Design review of the part built by this model. Coordinates are the model's own, in mm. A direction names the side the tool comes from. Give positions to 0.01 mm unless a question says otherwise; leave off trailing zeros. Loops run counter-clockwise (first coordinate to the right, second up) from the corner with the lowest first, then second, coordinate; pieces in that order, holes last. Notation, with made-up numbers: (36, 59.25) - (71, 59.25) arc R6 ccw to (71, 66.25) - close; hole circle Ø6 at (84.25, 89.5). An arc over 180 degrees is marked (long way). Put each result on its own line as item: value. Start each with the question number.
```python
from build123d import *

# Parameters (mm, degrees)
EXTRUDE_1_DEPTH     = 80
CUT_EXTRUDE_1_DEPTH = 40
EXTRUDE_2_DEPTH     = 40
SKETCH_5_R          = 21.930814163
SKETCH_5_R_2        = 25.847454044
EXTRUDE_3_DEPTH     = 30
SKETCH_6_R          = 10
EXTRUDE_4_DEPTH     = 20


with BuildPart() as part:
    # 草图2 → 凸台-拉伸1 (new body)
    with BuildSketch(Plane(origin=(0, 0, 0), x_dir=(0, 0, -1), z_dir=(1, 0, 0))):
        with BuildLine():
            Line((158.264812498, -105.800263885), (278.081233304, -38.403527181))
            ThreePointArc((278.081233304, -38.403527181), (294.118007975, -22.634152676), (300, -0.925779085))
            Line((300, -0.925779085), (300, 0.925779085))
            ThreePointArc((300, 0.925779085), (287.405591591, 31.331370676), (257, 43.925779085))
            Line((257, 43.925779085), (-257, 43.925779085))
            ThreePointArc((-257, 43.925779085), (-287.405591591, 31.331370676), (-300, 0.925779085))
            Line((-300, 0.925779085), (-300, -0.925779085))
            ThreePointArc((-300, -0.925779085), (-294.118007975, -22.634152676), (-278.081233304, -38.403527181))
            Line((-278.081233304, -38.403527181), (-158.264812498, -105.800263885))
            ThreePointArc((-158.264812498, -105.800263885), (-139.316019316, -113.463120111), (-119.043913327, -116.074220915))
            Line((-119.043913327, -116.074220915), (119.043913327, -116.074220915))
            ThreePointArc((119.043913327, -116.074220915), (139.316019316, -113.463120111), (158.264812498, -105.800263885))
        make_face()
    extrude(amount=EXTRUDE_1_DEPTH)

    # 草图3 → 切除-拉伸1 (cut)
    with BuildSketch(Plane(origin=(80, 0, 0), x_dir=(0, 0, -1), z_dir=(1, 0, 0))):
        with BuildLine():
            Line((257, 33.925779085), (-257, 33.925779085))
            ThreePointArc((-257, 33.925779085), (-280.334523779, 24.260302864), (-290, 0.925779085))
            Line((-290, 0.925779085), (-290, -0.925779085))
            ThreePointArc((-290, -0.925779085), (-285.485913097, -17.585693701), (-273.178620908, -29.68777181))
            Line((-273.178620908, -29.68777181), (-153.362200102, -97.084508514))
            ThreePointArc((-153.362200102, -97.084508514), (-136.782006067, -103.789507712), (-119.043913327, -106.074220915))
            Line((-119.043913327, -106.074220915), (119.043913327, -106.074220915))
            ThreePointArc((119.043913327, -106.074220915), (136.782006067, -103.789507712), (153.362200102, -97.084508514))
            Line((153.362200102, -97.084508514), (273.178620908, -29.68777181))
            ThreePointArc((273.178620908, -29.68777181), (285.485913097, -17.585693701), (290, -0.925779085))
            Line((290, -0.925779085), (290, 0.925779085))
            ThreePointArc((290, 0.925779085), (280.334523779, 24.260302864), (257, 33.925779085))
        make_face()
    extrude(amount=-CUT_EXTRUDE_1_DEPTH, mode=Mode.SUBTRACT)

    # 草图4 → 凸台-拉伸2 (add)
    with BuildSketch(Plane(origin=(40, 0, 0), x_dir=(0, 0, -1), z_dir=(1, 0, 0))):
        with BuildLine():
            Line((-237.264786543, 20.974123526), (-239.546765639, 17.833248756))
            ThreePointArc((-239.546765639, 17.833248756), (-236.865961455, 14.739716181), (-234.683185749, 11.276748513))
            Line((-234.683185749, 11.276748513), (-230.908435146, 12.503239332))
            Line((-230.908435146, 12.503239332), (-228.206060722, 4.186186056))
            Line((-228.206060722, 4.186186056), (-231.89838046, 2.986478649))
            ThreePointArc((-231.89838046, 2.986478649), (-231.547897142, -1.09197894), (-231.817475826, -5.176582004))
            Line((-231.817475826, -5.176582004), (-228.042725222, -6.403072824))
            Line((-228.042725222, -6.403072824), (-230.745099646, -14.720126099))
            Line((-230.745099646, -14.720126099), (-234.437419384, -13.520418692))
            ThreePointArc((-234.437419384, -13.520418692), (-236.551129646, -17.025969117), (-239.170092825, -20.172028037))
            Line((-239.170092825, -20.172028037), (-236.837168653, -23.383022689))
            Line((-236.837168653, -23.383022689), (-243.912076745, -28.5232443))
            Line((-243.912076745, -28.5232443), (-246.194055841, -25.38236953))
            ThreePointArc((-246.194055841, -25.38236953), (-249.964594205, -26.976011679), (-253.932586961, -27.981838877))
            Line((-253.932586961, -27.981838877), (-253.932586961, -31.950846543))
            Line((-253.932586961, -31.950846543), (-262.677654297, -31.950846543))
            Line((-262.677654297, -31.950846543), (-262.677654297, -28.068511818))
            ThreePointArc((-262.677654297, -28.068511818), (-266.664803265, -27.141528556), (-270.466187231, -25.62293223))
            Line((-270.466187231, -25.62293223), (-272.799111403, -28.833926882))
            Line((-272.799111403, -28.833926882), (-279.874019495, -23.693705272))
            Line((-279.874019495, -23.693705272), (-277.592040399, -20.552830502))
            ThreePointArc((-277.592040399, -20.552830502), (-280.272844583, -17.459297927), (-282.455620289, -13.996330258))
            Line((-282.455620289, -13.996330258), (-286.230370892, -15.222821078))
            Line((-286.230370892, -15.222821078), (-288.932745316, -6.905767802))
            Line((-288.932745316, -6.905767802), (-285.240425578, -5.706060395))
            ThreePointArc((-285.240425578, -5.706060395), (-285.590908896, -1.627602806), (-285.321330213, 2.457000258))
            Line((-285.321330213, 2.457000258), (-289.096080816, 3.683491078))
            Line((-289.096080816, 3.683491078), (-286.393706392, 12.000544353))
            Line((-286.393706392, 12.000544353), (-282.701386654, 10.800836946))
            ThreePointArc((-282.701386654, 10.800836946), (-280.587676392, 14.306387371), (-277.968713213, 17.452446291))
            Line((-277.968713213, 17.452446291), (-280.301637385, 20.663440943))
            Line((-280.301637385, 20.663440943), (-273.226729293, 25.803662554))
            Line((-273.226729293, 25.803662554), (-270.944750197, 22.662787784))
            ThreePointArc((-270.944750197, 22.662787784), (-267.174211833, 24.256429933), (-263.206219077, 25.262257132))
            Line((-263.206219077, 25.262257132), (-263.206219077, 29.231264797))
            Line((-263.206219077, 29.231264797), (-254.461151741, 29.231264797))
            Line((-254.461151741, 29.231264797), (-254.461151741, 25.348930073))
            ThreePointArc((-254.461151741, 25.348930073), (-250.474002773, 24.42194681), (-246.672618807, 22.903350484))
            Line((-246.672618807, 22.903350484), (-244.339694635, 26.114345136))
            Line((-244.339694635, 26.114345136), (-237.264786543, 20.974123526))
        make_face()
    extrude(amount=EXTRUDE_2_DEPTH)

    # 草图5 → 凸台-拉伸3 (add)
    with BuildSketch(Plane(origin=(40, 0, 0), x_dir=(0, 0, -1), z_dir=(1, 0, 0))):
        with Locations((-129.354117612, -82.245801831)):
            Circle(SKETCH_5_R)
        with Locations((-44.354117612, -82.245801831)):
            Circle(SKETCH_5_R)
        with Locations((40.645882388, -82.245801831)):
            Circle(SKETCH_5_R)
        with Locations((125.645882388, -82.245801831)):
            Circle(SKETCH_5_R)
        with Locations((258.847706699, 0)):
            Circle(SKETCH_5_R_2)
    extrude(amount=EXTRUDE_3_DEPTH)

    # 草图6 → 凸台-拉伸4 (add)
    with BuildSketch(Plane.ZY):
        with Locations((-180, -16.074220915)):
            Circle(SKETCH_6_R)
        with Locations((180, -16.074220915)):
            Circle(SKETCH_6_R)
    extrude(amount=EXTRUDE_4_DEPTH)


solid = part.part
```
Item 1: Machinability: for faces 1 (the flat face through (39, -116.074, 2)), 2 (the cylindrical face through (-9.86, -19.9, 189.24)), 3 (the cylindrical face through (60.28, -103.853, -136.539)), which of the approach directions +Z, -Z, +X, -X, +Y, -Y give a long, thin tool a straight path to every point of the face, cutting with its end or side? Answer none if there is none.
Item 2: For L1, parallel to Y at x = 70, z = 102; L2, parallel to Y at x = 57.5, z = 259; L3, parallel to Z at x = -9.5, y = -17.5, list the stretches that pass through material, from the lowest coordinate up. Write a range as from..to.
Item 3: Consider section B-B (z = -246). State the section outline as (x, y) points.
Item 4: Consider section C-C (y = -76). State the section outline as (x, z) points.
Item 5: Consider section A-A (x = 34). State the section outline as (y, z) points, plus the area to 3 significant figures.
Item 6: For P1, Ø4.5, axis at x = 63, z = 256.5, coming from the -Y side; P2, Ø1.5, axis at y = -7, z = -44.5, coming from the -X side; P3, Ø4.5, axis at x = 51, z = 260, coming from the +Y side, all flat-tipped, find the tip position at first contact; note any pin that passes through.
Item 7: Mouldability with a two-part tool opening along Z and no side actions: class faces 4 (the flat face through (39.44, -71.63, 219.01)), 5 (the flat face through (39.44, -72.574, -217.334)), 6 (the cylindrical face through (60.28, -103.725, 137.025)) as pulls with the +Z half, pulls with the -Z half, needs draft (parallel to the pull), parting line crosses it, or undercut.
Geometry says:
1. face 1: +Z, -Z, +X, -X, -Y
1. face 2: -X
1. face 3: +X
2. L1: y = -116.07..-106.07, 33.93..43.93
2. L2: y = -49.14..-37.66, -31.95..29.23, 33.87..43.88
2. L3: z = -189.9..-170.1, 170.1..189.9
3. outline: (0, -56.45) - (80, -56.45) - (80, -44.98) - (40, -44.98) - (40, -22.43) - (70, -22.43) - (70, 22.43) - (40, 22.43) - (40, 33.93) - (80, 33.93) - (80, 43.93) - (0, 43.93) - close
4. outline: (0, -211.24) - (80, -211.24) - (80, -190.85) - (40, -190.85) - (40, -146.67) - (70, -146.67) - (70, -104.62) - (40, -104.62) - (40, -61.67) - (70, -61.67) - (70, -19.62) - (40, -19.62) - (40, 23.33) - (70, 23.33) - (70, 65.38) - (40, 65.38) - (40, 108.33) - (70, 108.33) - (70, 150.38) - (40, 150.38) - (40, 190.85) - (80, 190.85) - (80, 211.24) - (0, 211.24) - close
5. outline: (-116.07, -119.04) arc R80 ccw to (-105.8, -158.26) - (-38.4, -278.08) arc R43 ccw to (-0.93, -300) - (0.93, -300) arc R43 ccw to (43.93, -257) - (43.93, 257) arc R43 ccw to (0.93, 300) - (-0.93, 300) arc R43 ccw to (-38.4, 278.08) - (-105.8, 158.26) arc R80 ccw to (-116.07, 119.04) - close
5. area: 80,500 mm2
6. P1: stops at y = -51.81
6. P2: stops at x = 0
6. P3: stops at y = 43.92
7. face 4: pulls with the +Z half
7. face 5: pulls with the -Z half
7. face 6: undercut
